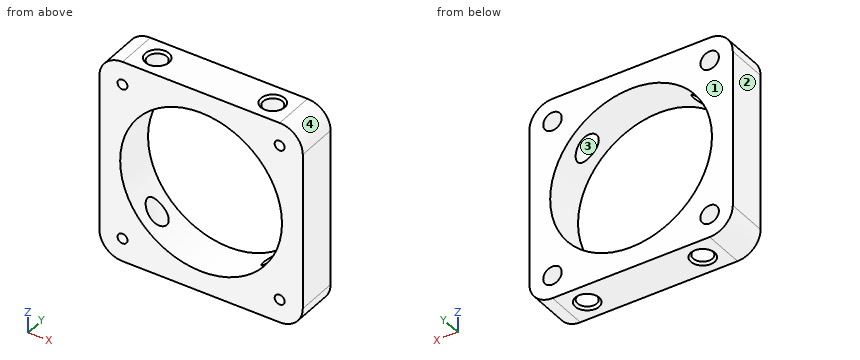
```python
from build123d import *

# Parameters (mm, degrees)
SKETCH1_W           = 88
SKETCH1_H           = 88
BOSS_EXTRUDE1_DEPTH = 18
FILLET1_R           = 10
SKETCH2_R           = 2.15
CUT_EXTRUDE1_DEPTH  = 19
SKETCH3_R           = 4.15
CUT_EXTRUDE2_DEPTH  = 89
SKETCH4_R           = 35
CUT_EXTRUDE3_DEPTH  = 19
CHAMFER1_SIZE       = 1
SKETCH5_R           = 4
CUT_EXTRUDE4_DEPTH  = 13


with BuildPart() as part:
    # Sketch1 → Boss-Extrude1 (new body)
    with BuildSketch(Plane(origin=(0, 0, 0), x_dir=(1, 0, 0), z_dir=(0, 1, 0))):
        Rectangle(SKETCH1_W, SKETCH1_H)
    extrude(amount=BOSS_EXTRUDE1_DEPTH)

    # Fillet1
    fillet1_edges = [part.edges().sort_by_distance(p)[0] for p in [
        (-44, 9, -44),
        (-44, 9, 44),
        (44, 9, 44),
        (44, 9, -44),
    ]]
    fillet(fillet1_edges, radius=FILLET1_R)

    # Sketch2 → Cut-Extrude1 (cut, through all)
    with BuildSketch(Plane(origin=(0, 18, 0), x_dir=(1, 0, 0), z_dir=(0, 1, 0))):
        with Locations((-34, 34)):
            Circle(SKETCH2_R)
        with Locations((34, 34)):
            Circle(SKETCH2_R)
        with Locations((34, -34)):
            Circle(SKETCH2_R)
        with Locations((-34, -34)):
            Circle(SKETCH2_R)
    extrude(amount=-CUT_EXTRUDE1_DEPTH, mode=Mode.SUBTRACT)

    # Sketch3 → Cut-Extrude2 (cut, through all)
    with BuildSketch(Plane.XY.offset(44)):
        with Locations((-25, 9)):
            Circle(SKETCH3_R)
        with Locations((25, 9)):
            Circle(SKETCH3_R)
    extrude(amount=-CUT_EXTRUDE2_DEPTH, mode=Mode.SUBTRACT)

    # Sketch4 → Cut-Extrude3 (cut, through all)
    with BuildSketch(Plane(origin=(0, 18, 0), x_dir=(1, 0, 0), z_dir=(0, 1, 0))):
        Circle(SKETCH4_R)
    extrude(amount=-CUT_EXTRUDE3_DEPTH, mode=Mode.SUBTRACT)

    # Chamfer1
    chamfer1_edges = [part.edges().sort_by_distance(p)[0] for p in [
        (-29.15, 9, -44),
        (-29.15, 9, 44),
        (20.85, 9, -44),
        (20.85, 9, 44),
    ]]
    chamfer(chamfer1_edges, length=CHAMFER1_SIZE)

    # Sketch5 → Cut-Extrude4 (cut)
    with BuildSketch(Plane(origin=(0, 18, 0), x_dir=(1, 0, 0), z_dir=(0, 1, 0))):
        with Locations((-34, 34)):
            Circle(SKETCH5_R)
        with Locations((34, 34)):
            Circle(SKETCH5_R)
        with Locations((34, -34)):
            Circle(SKETCH5_R)
        with Locations((-34, -34)):
            Circle(SKETCH5_R)
    extrude(amount=-CUT_EXTRUDE4_DEPTH, mode=Mode.SUBTRACT)


solid = part.part
```
Can you work these out from the model? Positions are in its coordinate system, mm. Face numbers are marked on the shaded views. Coordinates: 2 decimals unless noted, no trailing zeros. Loops run counter-clockwise (first coordinate to the right, second up) from the corner with the lowest first, then second, coordinate; pieces in that order, holes last.
Item 1: If we mould it in two halves opening along X, with no side actions, what happens to the marked faces 1, 2, 3 and 4? For each: released by +X, released by -X, zero draft, split by the parting line, or undercut.
Answers below:
face 1: zero draft
face 2: released by -X
face 3: undercut
face 4: released by +X
Item 2: Suppose I cut it at A-A (y = 1.75). Please give me the cut outline in (x, z).
Answers below:
outline: (-44, -34) arc R10 ccw to (-34, -44) - (34, -44) arc R10 ccw to (44, -34) - (44, 34) arc R10 ccw to (34, 44) - (-34, 44) arc R10 ccw to (-44, 34) - close; hole circle Ø4.3 at (-34, -34); hole circle Ø4.3 at (-34, 34); hole circle Ø70 at (0, 0); hole circle Ø4.3 at (34, -34); hole circle Ø4.3 at (34, 34)
Item 3: I'm going to push flat-ended pins straight in: pin 1 (9.5 mm diameter, centred on x = 25, y = 9, fed in from -Z); pin 2 (2.5 mm diameter, centred on x = 34.5, z = -35.5, fed in from +Y); pin 3 (12 mm diameter, centred on x = 7, z = -25, fed in from -Y); pin 4 (9.5 mm diameter, centred on x = -25, y = 9, fed in from +Z). Where does each tip first touch, or does it pass through?
Answers below:
pin 1: stops at z = -43.6
pin 2: stops at y = 5
pin 3: passes through
pin 4: stops at z = 43.6
Item 4: Please list where these lines run through material, in increasing order: L1, parallel to X at y = 4, z = 14.5; L2, parallel to X at y = 7.75, z = 37.5; L3, parallel to Y at x = -25, z = -33.5.
Answers below:
L1: x = -44 to -31.86, 31.86 to 44
L2: x = -43.37 to -35.94, -32.06 to -28.96, -21.04 to 21.04, 28.96 to 32.06, 35.94 to 43.37
L3: y = 0 to 4.85, 13.15 to 18
Item 5: Suppose I cut it at D-D (x = 25). Please give me the cut outline in (y, z).
Answers below:
outline: (0, -44) - (3.85, -44) - (4.85, -43) - (4.85, -24.49) - (0, -24.49) - close; (0, 24.49) - (4.85, 24.49) - (4.85, 43) - (3.85, 44) - (0, 44) - close; (13.15, -43) - (14.15, -44) - (18, -44) - (18, -24.49) - (13.15, -24.49) - close; (13.15, 24.49) - (18, 24.49) - (18, 44) - (14.15, 44) - (13.15, 43) - close
Item 6: Suppose I cut it at C-C (z = -6). Please give me the cut outline in (x, y).
Answers below:
outline: (-44, 0) - (-34.48, 0) - (-34.48, 18) - (-44, 18) - close; (34.48, 0) - (44, 0) - (44, 18) - (34.48, 18) - close
Item 7: Suppose I cut it at B-B (x = -18). Please give me the cut outline in (y, z).
Answers below:
outline: (0, -44) - (18, -44) - (18, -30.02) - (0, -30.02) - close; (0, 30.02) - (18, 30.02) - (18, 44) - (0, 44) - close
